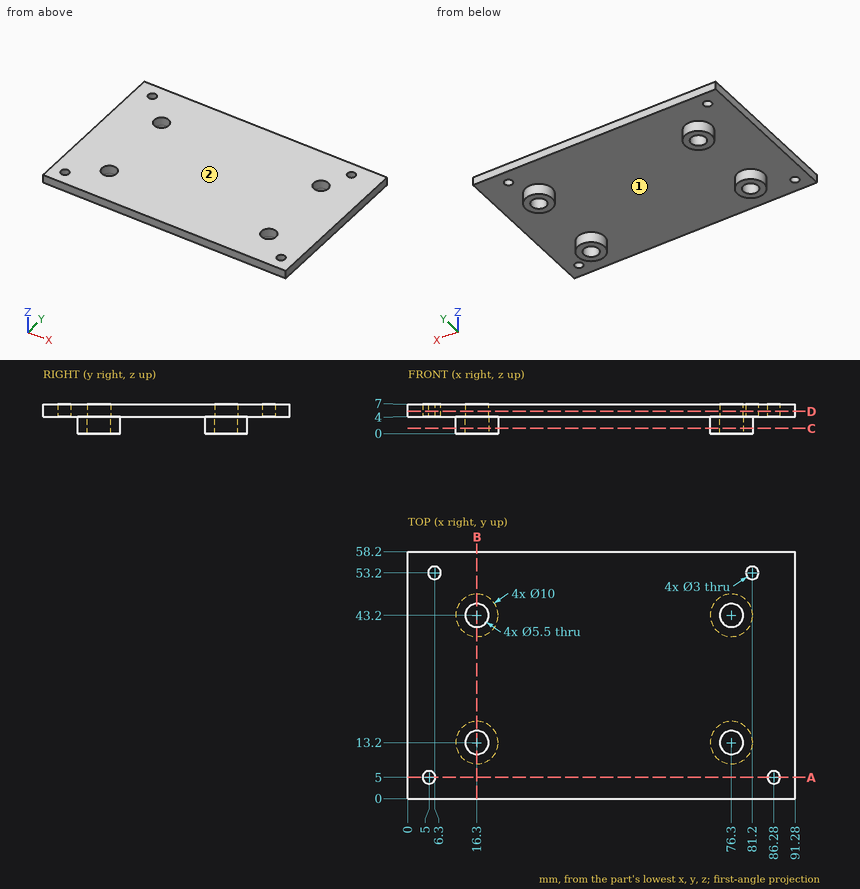
Print and shaded views of the part. All mm, measured from the part's lowest x, y and z. Give positions to 0.01 mm unless a question says otherwise; leave off trailing zeros. Loops run counter-clockwise (first coordinate to the right, second up) from the corner with the lowest first, then second, coordinate; pieces in that order, holes last. Notation, with made-up numbers: (-18.75, 41.5) -> (6.25, 41.5) arc R25 cw to (6.25, 54.5) -> close; hole circle Ø11 at (73, 57). An arc over 180 degrees is marked (long way). Use CSV: the item, a comma, the result in double quotes. Start each with the question number.
1) Flat gauge pin, fed straight in: pin 1 Ø1 at (x, y) = (52, 47) entering from -Z. Where does the tip first touch, or does it go through?
2) Mould opens along X. For the marked faces 1 and 2 say: released by +X, released by -X, zero draft, split by the parting line, or undercut.
3) Wall check: line 1 (Y direction, x = 16.3, z = 3.1); line 2 (Y direction, x = 76.3, z = 5.65); line 3 (Y direction, x = 86.28, z = 5.25). Give the ranges that are in metal, low to high.
4) Slice it at C-C on z = 1.25. Give the cut face in (x, y), plus the area to 3 significant figures.
5) Slice it at D-D on z = 5.25. Give the number of separate pieces and of enclosed holes in the cut face, plus the area to 3 significant figures.
6) Slice it at A-A on y = 5. Give the cut face in (x, z).
7) Slice it at B-B on x = 16.3. Give the cut face in (y, z).
Computed values:
1,pin 1,"stops at z = 4"
2,face 1,"undercut"
2,face 2,"zero draft"
3,line 1,"y = 8.2 to 10.45, 15.95 to 18.2, 38.2 to 40.45, 45.95 to 48.2"
3,line 2,"y = 0 to 10.45, 15.95 to 40.45, 45.95 to 58.2"
3,line 3,"y = 0 to 3.5, 6.5 to 58.2"
4,outline,"circle Ø10 at (16.3, 13.2); circle Ø10 at (16.3, 43.2); circle Ø10 at (76.3, 13.2); circle Ø10 at (76.3, 43.2); hole circle Ø5.5 at (16.3, 13.2); hole circle Ø5.5 at (16.3, 43.2); hole circle Ø5.5 at (76.3, 13.2); hole circle Ø5.5 at (76.3, 43.2)"
4,area,"219 mm^2"
5,separate pieces,"1"
5,enclosed holes,"8"
5,area,"5,190 mm^2"
6,outline,"(0, 4) -> (3.5, 4) -> (3.5, 7) -> (0, 7) -> close; (6.5, 4) -> (84.78, 4) -> (84.78, 7) -> (6.5, 7) -> close; (87.78, 4) -> (91.28, 4) -> (91.28, 7) -> (87.78, 7) -> close"
7,outline,"(0, 4) -> (8.2, 4) -> (8.2, 0) -> (10.45, 0) -> (10.45, 7) -> (0, 7) -> close; (15.95, 0) -> (18.2, 0) -> (18.2, 4) -> (38.2, 4) -> (38.2, 0) -> (40.45, 0) -> (40.45, 7) -> (15.95, 7) -> close; (45.95, 0) -> (48.2, 0) -> (48.2, 4) -> (58.2, 4) -> (58.2, 7) -> (45.95, 7) -> close"
